from build123d import *

# Parameters (mm, degrees)
SKETCH1_W           = 10
SKETCH1_H           = 250
BOSS_EXTRUDE1_DEPTH = 18
SHELL1_T            = -2
SKETCH3_R           = 5
CUT_EXTRUDE2_DEPTH  = 10
SKETCH4_R           = 5
CUT_EXTRUDE3_DEPTH  = 10
SKETCH5_W           = 18
SKETCH5_H           = 94
CUT_EXTRUDE4_DEPTH  = 10


with BuildPart() as part:
    # Sketch1 → Boss-Extrude1 (new body)
    with BuildSketch(Plane.XY):
        Rectangle(SKETCH1_W, SKETCH1_H)
    extrude(amount=BOSS_EXTRUDE1_DEPTH)

    # Shell1
    shell1_openings = [part.faces().sort_by_distance(p)[0] for p in [
        (0, 125, 9),
        (0, -125, 9),
    ]]
    offset(amount=SHELL1_T, openings=shell1_openings, kind=Kind.INTERSECTION)

    # Sketch3 → Cut-Extrude2 (cut)
    with BuildSketch(Plane.ZY.offset(5)):
        with Locations((9, -100)):
            Circle(SKETCH3_R)
    extrude(amount=-CUT_EXTRUDE2_DEPTH, mode=Mode.SUBTRACT)

    # Sketch4 → Cut-Extrude3 (cut)
    with BuildSketch(Plane(origin=(5, 0, 0), x_dir=(0, 0, -1), z_dir=(1, 0, 0))):
        with Locations((-9, -115)):
            Circle(SKETCH4_R)
    extrude(amount=-CUT_EXTRUDE3_DEPTH, mode=Mode.SUBTRACT)

    # Sketch5 → Cut-Extrude4 (cut)
    with BuildSketch(Plane(origin=(5, 0, 0), x_dir=(0, 0, -1), z_dir=(1, 0, 0))):
        with Locations((-9, 78)):
            Rectangle(SKETCH5_W, SKETCH5_H)
    extrude(amount=-CUT_EXTRUDE4_DEPTH, mode=Mode.SUBTRACT)


solid = part.part
Build history of the part. All positions in model axes, mm. A direction names the side the tool comes from. Round coordinates to 2 decimals unless told otherwise and drop trailing zeros. Loops run counter-clockwise (first coordinate to the right, second up) from the corner with the lowest first, then second, coordinate; pieces in that order, holes last. Notation, with made-up numbers: (-30.75, -9.75) -> (-0.75, -9.75) arc R22 ccw to (-0.75, 25.25) -> close; hole circle Ø9 at (-12.5, -6.5). An arc over 180 degrees is marked (long way). Use CSV: the item, a comma, the result in double quotes. Start each with the question number.
Q1. Saw through at B-B on x = 1. Give the cut face in (y, z).
Q2. Which spindle directions (+Z, -Z, +X, -X, +Y, -Y) get a long thin tool onto all of the face, cutting with end or side? Do faces 5 (the face through (0, -46, 16)), 6 (the face through (-4.01, -104.88, 7.92)). Say none if no direction does.
Q3. Saw through at A-A on y = -115. Give the cut face in (x, z), and give its area (3 significant figures).
Q4. Mould opens along X. For faces 1 (the face through (-5, -48, 9)), 2 (the face through (5, -48, 9)), 3 (the face through (3, -31, 9)), 4 (the face through (0, -46, 0)) say: +X half, -X half, draft (parallel to the pull), parting line (faces both ways), or undercut.
Q5. Saw through at D-D on y = -71. Give the cut face in (x, z), and give its area (3 significant figures).
Q6. Saw through at C-C on z = 7.5. Give the cut face in (x, y).
Q7. Drill centre lines: L1, parallel to Y at x = 3.85, z = 9; L2, parallel to X at y = -29, z = 11.75; L3, parallel to Z at x = 2.25, y = -51.5. Where is each one in solid material? Low to high.
Solutions:
1,outline,"(-125, 0) -> (31, 0) -> (31, 2) -> (-125, 2) -> close; (-125, 16) -> (31, 16) -> (31, 18) -> (-125, 18) -> close"
2,face 5,"+Y, -Y"
2,face 6,"+X, -X"
3,outline,"(-5, 0) -> (5, 0) -> (5, 4) -> (3, 4) -> (3, 2) -> (-3, 2) -> (-3, 4) -> (-5, 4) -> close; (-5, 14) -> (-3, 14) -> (-3, 16) -> (3, 16) -> (3, 14) -> (5, 14) -> (5, 18) -> (-5, 18) -> close"
3,area,"56.0 mm^2"
4,face 1,"-X half"
4,face 2,"+X half"
4,face 3,"undercut"
4,face 4,"draft"
5,outline,"(-5, 0) -> (5, 0) -> (5, 18) -> (-5, 18) -> close; hole (-3, 2) -> (3, 2) -> (3, 16) -> (-3, 16) -> close"
5,area,"96.0 mm^2"
6,outline,"(-5, -125) -> (-3, -125) -> (-3, -119.77) -> (-5, -119.77) -> close; (-5, -110.23) -> (-3, -110.23) -> (-3, -104.77) -> (-5, -104.77) -> close; (-5, -95.23) -> (-3, -95.23) -> (-3, 31) -> (-5, 31) -> close; (3, -125) -> (5, -125) -> (5, -119.77) -> (3, -119.77) -> close; (3, -110.23) -> (5, -110.23) -> (5, -104.77) -> (3, -104.77) -> close; (3, -95.23) -> (5, -95.23) -> (5, 31) -> (3, 31) -> close"
7,L1,"y = -125 to -120, -110 to -105, -95 to 31"
7,L2,"x = -5 to -3, 3 to 5"
7,L3,"z = 0 to 2, 16 to 18"
